Read the model definition and answer for the solid it produces. Units are mm, in the model's axes. A direction names the side the tool comes from. Round coordinates to 2 decimals unless told otherwise and drop trailing zeros. Order: outer loops, then holes, each group sorted by start corner. A loop starts at its lowest first (then second) coordinate and runs counter-clockwise, first axis right, second up. Notation, with made-up numbers: (-15.75, 26.5) -> (26.25, 26.5) arc R15 cw to (26.25, 50.5) -> close; hole circle Ø3 at (35, 25). An arc over 180 degrees is marked (long way). Answer as a JSON object with one key per item and string values. Group by question number.
Item 1: Section D-D, the plane x = 102 is taken. Write down the section's boundary in (y, z), plus the area to 3 significant figures.
Item 2: Section B-B, the plane z = 15 is taken. Write down the section's boundary in (x, y).
Item 3: For faces 1 (the flat face through (4, 190.5, 10)), 2 (the cylindrical face through (132.75, 171.18, 22.4)), determine the directions among +Z, -Z, +X, -X, +Y, -Y from which every point of the face is accessible in a straight line to the end or side of a thin tool.
Item 4: Section A-A, the plane x = 126 is taken. Write down the section's boundary in (y, z), plus the area to 3 significant figures.
Item 5: Section C-C, the plane z = 34.5 is taken. Write down the section's boundary in (x, y).
Item 6: The mould has two halves that part along X. Classify faces 3 (the flat face through (130, 190.5, 10)), 4 (the flat face through (-31.328, 75, 41)), 5 (the cylindrical face through (6.299, 171.183, 21.853)): pulls with the +X half, pulls with the -X half, needs draft (parallel to the pull), parting line crosses it, or undercut.
Item 7: Consider probe 1 along Y at (x, z) = (150.5, 70); probe 2 along X at (y, z) = (156, -0.5); probe 3 along Z at (x, y) = (12, 179.5). Determine where each line is inside the solid, lowest interval first. Write a range as from..to.
Autodesk Fusion 360 part; units mm, degrees
sketch "Sketch1" plane through (0, 0, 0) normal (0, 1, 0) x (1, 0, 0)
  line L0 (-31.3279, 23.8092) -> (159.1721, 23.8092)
  line L1 (159.1721, 23.8092) -> (159.1721, -103.1908)
  line L2 (159.1721, -103.1908) -> (-31.3279, -103.1908)
  line L3 (-31.3279, -103.1908) -> (-31.3279, 23.8092)
  dimension "d1" = 190.5
  dimension "d2" = 127
extrude "Extrude1" add sketch "Sketch1" along normal blind 152.4
sketch "Sketch2" plane through (0, 152.4, 0) normal (0, 1, 0) x (-1, 0, 0)
  line L0 (31.3279, 103.1908) -> (-159.1721, 103.1908)
  line L1 (-159.1721, 103.1908) -> (-159.1721, -23.8092)
  line L2 (-159.1721, -23.8092) -> (31.3279, -23.8092)
  line L3 (31.3279, -23.8092) -> (31.3279, 103.1908)
  circle A0 centre (-3.5457, 9.4553) radius 12.7
  circle A1 centre (-130, 10) radius 12.7
  dimension "d5" = 25.4
  dimension "d6" = 25.4
extrude "Extrude2" add sketch "Sketch2" along normal blind 38.1 contours A0
extrude "Extrude3" add sketch "Sketch2" along normal blind 38.1 contours A1
Values found:
{
 "1": {"outline": "(0, -23.81) -> (152.4, -23.81) -> (152.4, 103.19) -> (0, 103.19) -> close", "area": "19,400 mm2"},
 "2": {"outline": "(-31.33, 0) -> (159.17, 0) -> (159.17, 152.4) -> (141.67, 152.4) -> (141.67, 190.5) -> (118.33, 190.5) -> (118.33, 152.4) -> (14.97, 152.4) -> (14.97, 190.5) -> (-7.88, 190.5) -> (-7.88, 152.4) -> (-31.33, 152.4) -> close"},
 "3": {"face 1": "+Z, -Z, +X, -X, +Y", "face 2": "+Y"},
 "4": {"outline": "(0, -23.81) -> (152.4, -23.81) -> (152.4, -2.05) -> (190.5, -2.05) -> (190.5, 22.05) -> (152.4, 22.05) -> (152.4, 103.19) -> (0, 103.19) -> close", "area": "20,300 mm2"},
 "5": {"outline": "(-31.33, 0) -> (159.17, 0) -> (159.17, 152.4) -> (-31.33, 152.4) -> close"},
 "6": {"face 3": "needs draft", "face 4": "pulls with the -X half", "face 5": "undercut"},
 "7": {"probe 1": "0..152.4", "probe 2": "-4.34..11.43, 122.86..137.14", "probe 3": "-0.02..18.93"}
}
